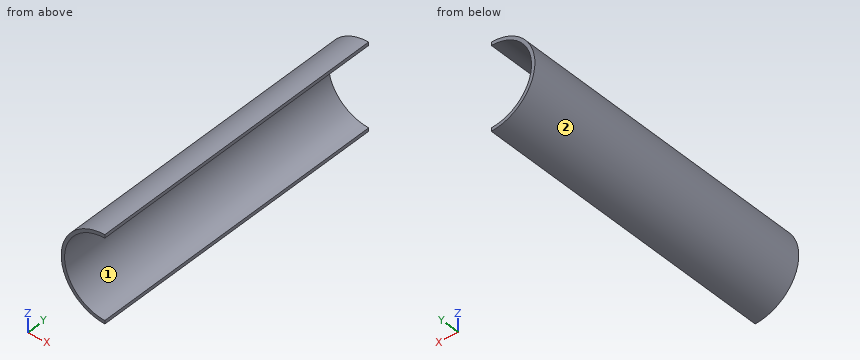
from build123d import *

# Parameters (mm, degrees)
SKETCH1_R           = 38.75
BOSS_EXTRUDE2_DEPTH = 270
CUT_EXTRUDE2_DEPTH  = 480
SKETCH4_W           = 38.75
SKETCH4_H           = 77.5
CUT_EXTRUDE3_DEPTH  = 480


with BuildPart() as part:
    # Sketch1 → Boss-Extrude2 (new body)
    with BuildSketch(Plane(origin=(0, 0, 0), x_dir=(1, 0, 0), z_dir=(0, 1, 0))):
        with Locations(Location((0, 0, 0), (0, 0, 270))):
            Circle(SKETCH1_R)
    extrude(amount=BOSS_EXTRUDE2_DEPTH)

    # Sketch3 → Cut-Extrude2 (cut)
    with BuildSketch(Plane(origin=(0, 270, 0), x_dir=(1, 0, 0), z_dir=(0, 1, 0))):
        with BuildLine():
            Line((0, -35.75), (0, 35.75))
            ThreePointArc((0, 35.75), (-35.75, 0), (0, -35.75))
        make_face()
    extrude(amount=-CUT_EXTRUDE2_DEPTH, mode=Mode.SUBTRACT)

    # Sketch4 → Cut-Extrude3 (cut)
    with BuildSketch(Plane(origin=(0, 270, 0), x_dir=(1, 0, 0), z_dir=(0, 1, 0))):
        with Locations((19.375, 0)):
            Rectangle(SKETCH4_W, SKETCH4_H)
    extrude(amount=-CUT_EXTRUDE3_DEPTH, mode=Mode.SUBTRACT)


solid = part.part
Here's how the part is built. I have some questions about the finished solid (model axes, mm). Face numbers are marked on the shaded views. Give positions to 0.01 mm unless a question says otherwise; leave off trailing zeros. Order: outer loops, then holes, each group sorted by start corner. A loop starts at its lowest first (then second) coordinate and runs counter-clockwise, first axis right, second up. Notation, with made-up numbers: (74, 76) -> (80, 76) arc R19 ccw to (80, 103) -> close; hole circle Ø9 at (42.25, 3). An arc over 180 degrees is marked (long way). Use a Markdown table: item, result. Add a question column.
Item 1: Imagine slicing it at A-A on x = -28. Please give me the cut outline in (y, z), plus the area to 3 significant figures.
Item 2: Imagine slicing it at C-C on y = 68. Please give me the cut outline in (x, z), plus the area to 3 significant figures.
Item 3: I need wall thicknesses on line 1 (Z direction, x = -32.5, y = 63); line 2 (Z direction, x = -33, y = 131.5); line 3 (X direction, y = 93.5, z = 3.5). Which ranges of each line are inside material? Lowest first, please.
Item 4: Will these pins go through, and if not, where does the flat tip stop? pin 1 (12 mm diameter, centred on x = -10.5, z = 23.5, fed in from -Y); pin 2 (6 mm diameter, centred on x = -7.5, y = 216.5, fed in from +Z); pin 3 (10 mm diameter, centred on y = 56.5, z = -30.5, fed in from -X); pin 4 (2 mm diameter, centred on y = 159, z = 28.5, fed in from +X).
Item 5: Imagine slicing it at B-B on z = 0. Please give me the cut outline in (x, y).
Item 6: If we mould it in two halves opening along Z, with no side actions, what happens to the marked faces 1 and 2? For each: pulls with the +Z half, pulls with the -Z half, needs draft (parallel to the pull), parting line crosses it, or undercut.
Data:
| question | item | result |
|---|---|---|
| 1 | outline | (0, -26.79) -> (270, -26.79) -> (270, -22.23) -> (0, -22.23) -> close; (0, 22.23) -> (270, 22.23) -> (270, 26.79) -> (0, 26.79) -> close |
| 1 | area | 2,460 mm² |
| 2 | outline | (0, -38.75) -> (0, -35.75) arc R35.75 cw to (0, 35.75) -> (0, 38.75) arc R38.75 ccw to start |
| 2 | area | 351 mm² |
| 3 | line 1 | z = -21.1 to -14.89, 14.89 to 21.1 |
| 3 | line 2 | z = -20.31 to -13.75, 13.75 to 20.31 |
| 3 | line 3 | x = -38.59 to -35.58 |
| 4 | pin 1 | passes through |
| 4 | pin 2 | stops at z = 38.49 |
| 4 | pin 3 | stops at x = -29.18 |
| 4 | pin 4 | stops at x = -20.19 |
| 5 | outline | (-38.75, 0) -> (-35.75, 0) -> (-35.75, 270) -> (-38.75, 270) -> close |
| 6 | face 1 | undercut |
| 6 | face 2 | parting line crosses it |
